Build history of the part. All positions in model axes, mm. A direction names the side the tool comes from. Round coordinates to 2 decimals unless told otherwise and drop trailing zeros. Order: outer loops, then holes, each group sorted by start corner. A loop starts at its lowest first (then second) coordinate and runs counter-clockwise, first axis right, second up. Notation, with made-up numbers: M 84.5,-32.5 L 128.5,-32.5 A16 cw 128.5,-16.5 Z; hole C 56.5,-38.75 d2. An arc over 180 degrees is marked long. Use CSV: the item, a comma, the result in double quotes.
from build123d import *

# Parameters (mm, degrees)
SKETCH_1_R           = 67.5
EXTRUDE_1_DEPTH      = 5
SKETCH_2_W           = 6
SKETCH_2_H           = 35
EXTRUDE_2_DEPTH      = 60
FILLET_1_R           = 17.5
SKETCH_3_R           = 16
CUT_EXTRUDE_1_DEPTH  = 5
CHAMFER_1_SIZE       = 1.640243073
CHAMFER_1_SIZE_2     = 0.8
SKETCH_4_R           = 15
CUT_EXTRUDE_2_DEPTH  = 121.188675061
SKETCH_6_W           = 2
SKETCH_6_H           = 6
CUT_EXTRUDE_3_DEPTH  = 121.817372977
SKETCH_8_R           = 1.6
CUT_EXTRUDE_5_DEPTH  = 6
CUT_EXTRUDE_START    = -2
CUT_EXTRUDE_8_DEPTH  = 2.2
SKETCH_11_W          = 25
SKETCH_11_H          = 10.5
EXTRUDE_4_DEPTH      = 7.3
EXTRUDE_5_DEPTH      = 2
FILLET_3_R           = 1
EXTRUDE_6_DEPTH      = 5
SKETCH_14_R          = 1.15
CUT_EXTRUDE_10_DEPTH = 127.019830237
FILLET_2_R           = 0.5
SKETCH_15_R          = 2
CUT_EXTRUDE_11_DEPTH = 10
SKETCH_16_W          = 56.328401117
SKETCH_16_H          = 65
CUT_EXTRUDE_12_DEPTH = 2
SKETCH_17_W          = 112.249721604
SKETCH_17_H          = 30
CUT_EXTRUDE_13_DEPTH = 113.749722891


# Some blends are built 0.0001 mm under size
with BuildPart() as part:
    # 스케치1 → 보스-돌출1 (new body)
    with BuildSketch(Plane(origin=(0, 0, 0), x_dir=(1, 0, 0), z_dir=(0, 1, 0))):
        with Locations(Location((0, 0, 0), (0, 0, 270))):
            Circle(SKETCH_1_R)
    extrude(amount=EXTRUDE_1_DEPTH)

    # 스케치2 → 보스-돌출2 (add)
    with BuildSketch(Plane(origin=(0, 5, 0), x_dir=(1, 0, 0), z_dir=(0, 1, 0))):
        with Locations((5.76, -20)):
            Rectangle(SKETCH_2_W, SKETCH_2_H)
    extrude(amount=EXTRUDE_2_DEPTH)

    # 필렛1
    fillet_1_edges = [part.edges().sort_by_distance(p)[0] for p in [
        (5.76, 65, 2.5),
        (5.76, 65, 37.5),
    ]]
    fillet(fillet_1_edges, radius=FILLET_1_R - 0.0001)  # a hair under: the kernel refuses the full size

    # 스케치3 → 컷-돌출1 (cut)
    with BuildSketch(Plane.ZY.offset(-2.76)):
        with Locations((20, 47.5)):
            Circle(SKETCH_3_R)
    extrude(amount=-CUT_EXTRUDE_1_DEPTH, mode=Mode.SUBTRACT)

    # 모따기1
    # the kernel refuses this chamfer: 1.640243073, 0.8 mm, written as the material it takes off along each edge
    with BuildSketch(Plane(origin=(2.76, 47.5, 20), x_dir=(0, 0, 1), z_dir=(0, -1, 0))) as chamfer_1_piece_1:
        Polygon((16 + CHAMFER_1_SIZE, 0), (16, -CHAMFER_1_SIZE_2), (16, 0), align=None)
    revolve(axis=Axis((2.76, 47.5, 20), (-1, 0, 0)), mode=Mode.SUBTRACT)

    # 스케치4 → 컷-돌출2 (cut, through all)
    with BuildSketch(Plane.ZY.offset(-7.76)):
        with Locations((20, 47.5)):
            Circle(SKETCH_4_R)
    extrude(amount=-CUT_EXTRUDE_2_DEPTH, mode=Mode.SUBTRACT)

    # 스케치6 → 컷-돌출3 (cut, through all)
    with BuildSketch(Plane(origin=(8.76, 0, 0), x_dir=(0, 0, -1), z_dir=(1, 0, 0))):
        with Locations((-3.5, 24.5)):
            Rectangle(SKETCH_6_W, SKETCH_6_H)
    extrude(amount=-CUT_EXTRUDE_3_DEPTH, mode=Mode.SUBTRACT)

    # 스케치8 → 컷-돌출5 (cut)
    with BuildSketch(Plane(origin=(0, 0, 4.5), x_dir=(-1, 0, 0), z_dir=(0, 0, -1))):
        with Locations((-5.76, 24.5)):
            Circle(SKETCH_8_R)
    extrude(amount=-CUT_EXTRUDE_5_DEPTH, mode=Mode.SUBTRACT)

    # 스케치9 → 컷-돌출8 (cut)
    with BuildSketch(Plane(origin=(0, 0, 4.5), x_dir=(-1, 0, 0), z_dir=(0, 0, -1)).offset(CUT_EXTRUDE_START)):
        Polygon((-4.316624327, 27), (-7.203375673, 27), (-8.646751346, 24.5), (-7.203375673, 22), (-4.316624327, 22), (-2.76, 22), (-2.76, 27), align=None)
    extrude(amount=-CUT_EXTRUDE_8_DEPTH, mode=Mode.SUBTRACT)

    # 스케치11 → 보스-돌출4 (add)
    with BuildSketch(Plane(origin=(0, 5, 0), x_dir=(1, 0, 0), z_dir=(0, 1, 0))):
        with Locations((24.26, -7.75)):
            Rectangle(SKETCH_11_W, SKETCH_11_H)
        with Locations((24.26, -32.25)):
            Rectangle(SKETCH_11_W, SKETCH_11_H)
    extrude(amount=EXTRUDE_4_DEPTH)

    # 스케치12 → 보스-돌출5 (add)
    with BuildSketch(Plane(origin=(0, 12.3, 0), x_dir=(1, 0, 0), z_dir=(0, 1, 0))):
        Polygon((16.76, -32.5), (36.76, -32.5), (36.76, -37.5), (11.76, -37.5), (11.76, -27), (16.76, -27), align=None)
        Polygon((11.76, -2.5), (36.76, -2.5), (36.76, -7.5), (16.76, -7.5), (16.76, -13), (11.76, -13), align=None)
    extrude(amount=EXTRUDE_5_DEPTH)

    # 필렛3
    fillet_3_edges = [part.edges().sort_by_distance(p)[0] for p in [
        (36.76, 9.65, 2.5),
        (36.76, 9.65, 37.5),
        (36.76, 8.65, 27),
        (36.76, 8.65, 13),
    ]]
    fillet(fillet_3_edges, radius=FILLET_3_R)

    # 스케치13 → 보스-돌출6 (add)
    with BuildSketch(Plane(origin=(16.76, 0, 0), x_dir=(0, 0, -1), z_dir=(1, 0, 0))):
        with BuildLine():
            Line((-27, 14.3), (-37.5, 14.3))
            Line((-37.5, 14.3), (-37.5, 44.3))
            Line((-37.5, 44.3), (-30.524257694, 44.3))
            ThreePointArc((-30.524257694, 44.3), (-29.151964364, 41.397414624), (-27, 39.014718626))
            Line((-27, 39.014718626), (-27, 14.3))
        make_face()
        with BuildLine():
            Line((-13, 14.3), (-2.5, 14.3))
            Line((-2.5, 14.3), (-2.5, 44.3))
            Line((-2.5, 44.3), (-9.475742306, 44.3))
            ThreePointArc((-9.475742306, 44.3), (-10.848035636, 41.397414624), (-13, 39.014718626))
            Line((-13, 39.014718626), (-13, 14.3))
        make_face()
    extrude(amount=-EXTRUDE_6_DEPTH)

    # 스케치14 → 컷-돌출10 (cut, through all)
    with BuildSketch(Plane(origin=(16.76, 0, 0), x_dir=(0, 0, -1), z_dir=(1, 0, 0))):
        with Locations((-30.25, 18.3)):
            Circle(SKETCH_14_R)
        with Locations((-9.75, 18.3)):
            Circle(SKETCH_14_R)
        with Locations((-9.75, 38.8)):
            Circle(SKETCH_14_R)
        with Locations((-30.25, 38.8)):
            Circle(SKETCH_14_R)
    extrude(amount=-CUT_EXTRUDE_10_DEPTH, mode=Mode.SUBTRACT)

    # 필렛2
    fillet_2_edges = [part.edges().sort_by_distance(p)[0] for p in [
        (26.26, 12.3, 13),
        (16.76, 25.657359313, 13),
        (26.76, 12.3, 7.5),
        (36.76, 13.3, 7.5),
        (36.76, 12.3, 30.25),
        (16.76, 25.657359313, 27),
        (26.76, 12.3, 32.5),
        (36.76, 13.3, 32.5),
        (26.26, 12.3, 27),
        (36.467106781, 12.3, 27.292893219),
        (36.76, 12.3, 9.75),
        (36.467106781, 12.3, 12.707106781),
    ]]
    fillet(fillet_2_edges, radius=FILLET_2_R)

    # 스케치15 → 컷-돌출11 (cut)
    with BuildSketch(Plane.ZY.offset(-2.76)):
        with Locations((9.75, 38.8)):
            Circle(SKETCH_15_R)
        with Locations((30.25, 38.8)):
            Circle(SKETCH_15_R)
        with Locations((9.75, 18.3)):
            Circle(SKETCH_15_R)
        with Locations((30.25, 18.3)):
            Circle(SKETCH_15_R)
    extrude(amount=-CUT_EXTRUDE_11_DEPTH, mode=Mode.SUBTRACT)

    # 스케치16 → 컷-돌출12 (cut)
    with BuildSketch(Plane(origin=(0, 5, 0), x_dir=(1, 0, 0), z_dir=(0, 1, 0))):
        with Locations((-39.335799442, -35)):
            Rectangle(SKETCH_16_W, SKETCH_16_H)
    extrude(amount=-CUT_EXTRUDE_12_DEPTH, mode=Mode.SUBTRACT)

    # 스케치17 → 컷-돌출13 (cut, through all)
    with BuildSketch(Plane(origin=(0, 5, 0), x_dir=(1, 0, 0), z_dir=(0, 1, 0))):
        with Locations((0, -52.5)):
            Rectangle(SKETCH_17_W, SKETCH_17_H)
    extrude(amount=-CUT_EXTRUDE_13_DEPTH, mode=Mode.SUBTRACT)


solid = part.part
(1) Cut at C-C, the plane x = -16.5. Give the cut face in (y, z).
Answer block:
outline,"M 0,-65.45 L 5,-65.45 L 5,2.5 L 3,2.5 L 3,37.5 L 0,37.5 Z"
(2) Tool access for faces 1 (the face through (16, 15, 27)), 2 (the face through (27, 14.3, 5)), 3 (the face through (2.76, 20, 20)): list every direction of +Z, -Z, +X, -X, +Y, -Y with a clear straight run to the whole face (end or side of a thin tool).
Answer block:
face 1,"+X, +Y"
face 2,"+Z, -Z, +X, +Y"
face 3,"+Z, -Z, -X, +Y"
(3) Cut at A-A, the plane y = 8. Give the cut face in (x, z).
Answer block:
outline,"M 2.76,2.5 L 8.76,2.5 L 8.76,37.5 L 2.76,37.5 Z; M 11.76,2.5 L 35.76,2.5 A1 ccw 36.76,3.5 L 36.76,12 A1 ccw 35.76,13 L 11.76,13 Z; M 11.76,27 L 35.76,27 A1 ccw 36.76,28 L 36.76,36.5 A1 ccw 35.76,37.5 L 11.76,37.5 Z"
(4) Two-plate mould, pull along X, no slides. Class faces 4 (the face through (8.76, 28, 20)), 5 (the face through (2.04, 2.46, -67.47)), 6 (the face through (7, 26, 4.5)): released by +X, released by -X, zero draft, split by the parting line, or undercut.
Answer block:
face 4,"undercut"
face 5,"split by the parting line"
face 6,"zero draft"
(5) Cut at B-B, the plane z = 0. Give the cut face in (x, y).
Answer block:
outline,"M -67.5,0 L 67.5,0 L 67.5,5 L -67.5,5 Z"
(6) Drop flat-ended pins along their axis: pin 1 (10 mm diameter, centred on x = 41, z = -12, fed in from +Y); pin 2 (5.5 mm diameter, centred on x = 28, z = 36, fed in from +Y); pin 3 (1.2 mm diameter, centred on x = 27.5, y = 13.5, fed in from -Z); pin 4 (3 mm diameter, centred on x = -22.5, z = -47, fed in from -Y). Give the stop position or say it passes through.
Answer block:
pin 1,"stops at y = 5"
pin 2,"stops at y = 14.3"
pin 3,"stops at z = 2.5"
pin 4,"stops at y = 0"
(7) Wall check: line 1 (Z direction, x = 5, y = 18); line 2 (X direction, y = 27, z = 6); line 3 (Y direction, x = 6.3, z = 9.75). Give the ranges that are in metal, low to high. Write a range as from..to.
Answer block:
line 1,"z = 2.5..7.77, 11.73..28.27, 32.23..37.5"
line 2,"x = 2.76..8.76, 11.76..16.76"
line 3,"y = 0..16.3, 20.3..22.99, 26.01..35.21, 59.79..61.68"
(8) Cut at D-D, the plane x = 25. Give the cut face in (y, z), and give its area (3 significant figures).
Answer block:
outline,"M 0,-62.7 L 5,-62.7 L 5,2.5 L 14.3,2.5 L 14.3,7.5 L 12.8,7.5 A0.5 cw 12.3,8 L 12.3,12.5 A0.5 ccw 11.8,13 L 5,13 L 5,27 L 11.8,27 A0.5 ccw 12.3,27.5 L 12.3,32 A0.5 cw 12.8,32.5 L 14.3,32.5 L 14.3,37.5 L 0,37.5 Z"
area,"674 mm²"
